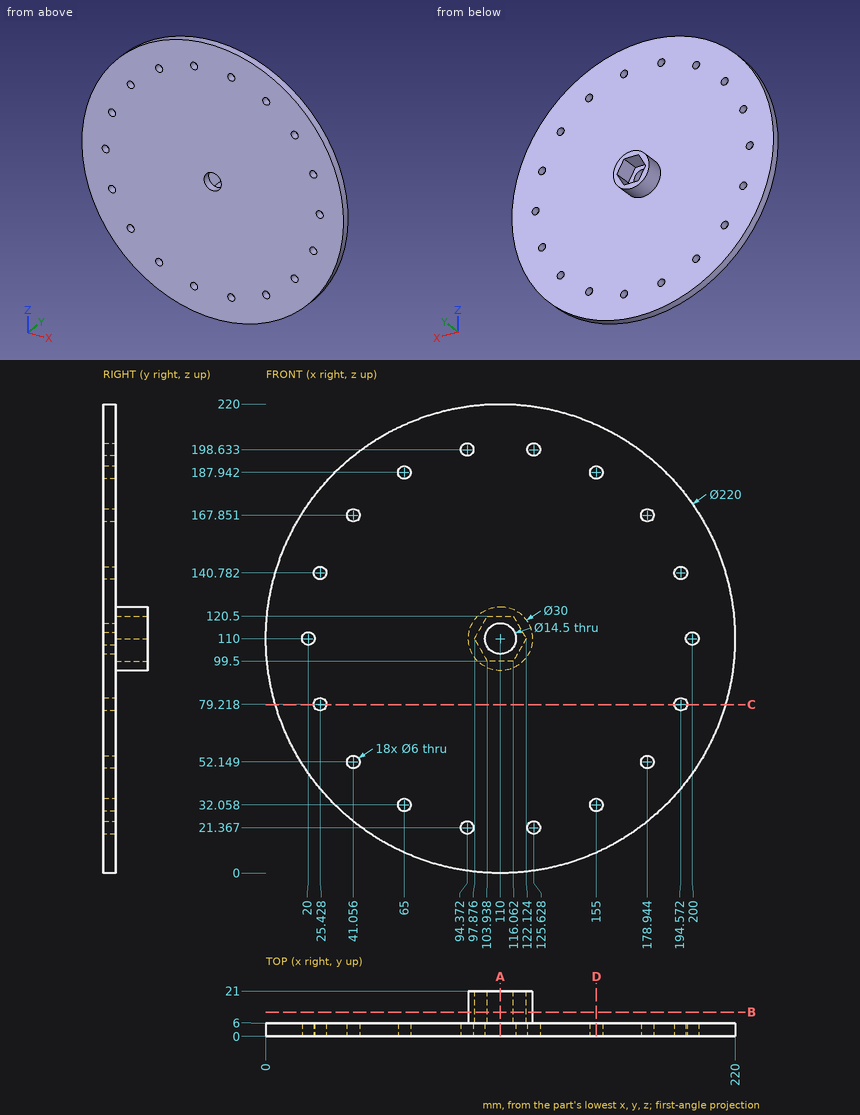
For this review, use the dimensioned drawing (mm, ordinates from the lowest corner) and the shaded views. Give positions to 0.01 mm unless a question says otherwise; leave off trailing zeros. Order: outer loops, then holes, each group sorted by start corner. A loop starts at its lowest first (then second) coordinate and runs counter-clockwise, first axis right, second up. Notation, with made-up numbers: (19.5, 83) -> (78.5, 83) arc R22 ccw to (78.5, 120) -> close; hole circle Ø8 at (-24, -34). An arc over 180 degrees is marked (long way). Write item = value, one per line. Start each with the question number.
(1) Take a section at D-D (x = 155). Write out the cut boundary in (y, z) (1 decimal).
(2) Take a section at A-A (x = 110). Write out the cut boundary in (y, z).
(3) Take a section at B-B (y = 11.25). Write out the cut boundary in (x, z) (1 decimal).
(4) For L1, parallel to X at y = 4, z = 30 (1 decimal); L2, parallel to X at y = 1.25, z = 110; L3, parallel to Y at x = 127.5, z = 172, list the stretches that pass through material, from the lowest coordinate up. Write a range as from..to.
(5) For pin 1 Ø8 at (x, z) = (200, 110) entering from +Y; pin 2 Ø5.5 at (x, z) = (94.37, 198.63) entering from +Y; pin 3 Ø8 at (y, z) = (8, 76.5) entering from -X; pin 4 Ø6 at (x, y) = (108.5, 12) entering from +Z, all flat-tipped, find the tip position at first contact; note any pin that passes through.
(6) Take a section at C-C (z = 79). Write out the cut boundary in (x, y) (1 decimal).
Returned:
q1.outline = (0, 9.6) -> (6, 9.6) -> (6, 29.1) -> (0, 29.1) -> close; (0, 35.1) -> (6, 35.1) -> (6, 184.9) -> (0, 184.9) -> close; (0, 190.9) -> (6, 190.9) -> (6, 210.4) -> (0, 210.4) -> close
q2.outline = (0, 0) -> (6, 0) -> (6, 95) -> (21, 95) -> (21, 99.5) -> (6, 99.5) -> (6, 102.75) -> (0, 102.75) -> close; (0, 117.25) -> (6, 117.25) -> (6, 120.5) -> (21, 120.5) -> (21, 125) -> (6, 125) -> (6, 220) -> (0, 220) -> close
q3.outline = circle Ø30 at (110, 110); hole (97.9, 110) -> (103.9, 99.5) -> (116.1, 99.5) -> (122.1, 110) -> (116.1, 120.5) -> (103.9, 120.5) -> close
q4.L1 = 34.5..62.8, 67.2..152.8, 157.2..185.5
q4.L2 = 0..17, 23..102.75, 117.25..197, 203..220
q4.L3 = 0..6
q5.pin_1 = 6
q5.pin_2 = through
q5.pin_3 = 4.18
q5.pin_4 = 125
q6.outline = (4.5, 0) -> (22.4, 0) -> (22.4, 6) -> (4.5, 6) -> close; (28.4, 0) -> (191.6, 0) -> (191.6, 6) -> (28.4, 6) -> close; (197.6, 0) -> (215.5, 0) -> (215.5, 6) -> (197.6, 6) -> close
